Work out the finished part from the listing and answer in its coordinate system (mm). A direction names the side the tool comes from. Coordinates: 2 decimals unless noted, no trailing zeros. Order: outer loops, then holes, each group sorted by start corner. A loop starts at its lowest first (then second) coordinate and runs counter-clockwise, first axis right, second up.
1. The part is cut by section C-C, the plane x = -35.5. Give the vertices of the cut face in (y, z).
2. Determine the mould class of faces 5 (the flat face through (-2, -476.179, 214)), 6 (the flat face through (-512.899, -98, 84)), 7 (the flat face through (-12, 489, 215.9)) for opening direction Y: +Y half, -Y half, draft (parallel to the pull), parting line (faces both ways), or undercut.
3. The part is cut by section B-B, the plane z = 109. Give the vertices of the cut face in (x, y).
4. Find the intervals of material crossed by probe 1 along Y at (x, z) = (298, 173); probe 2 along Y at (x, z) = (453.5, 57); probe 3 along X at (y, z) = (373, 88.5), in increasing order.
5. Flat-ended cylindrical pins translate along their axes: pin 1 Ø5 at (x, z) = (365.5, 160) entering from +Y; pin 2 Ø3 at (x, y) = (162, 30.5) entering from -Z. Find the tip coordinate at first contact, or state that the pin passes through.
6. The part is cut by section D-D, the plane z = 12. Give the vertices of the cut face in (x, y), then the cut area to 3 significant figures.
7. The part is cut by section A-A, the plane y = 359. Give the vertices of the cut face in (x, z), then the cut area to 3 significant figures.
8. A tool of negligible diameter and unlimited length cuts with its end or side. For faces 1 (the flat face through (2, 463.621, 91)), 2 (the flat face through (-12, -399.979, 126)), 3 (the flat face through (-12, 38.171, 132)), 4 (the flat face through (-12, 25.471, 126)), from which of +Z, -Z, +X, -X, +Y, -Y can it reach the whole face along a straight path? Write none if from no direction.
```python
from build123d import *

# Parameters (mm, degrees)
SKETCH1_W            = 1016
SKETCH1_H            = 412.75
BOSS_EXTRUDE2_DEPTH  = 203.2
SKETCH3_W            = 1041.4
SKETCH3_H            = 939.8
BOSS_EXTRUDE4_DEPTH  = 25.4
SKETCH6_W            = 12.7
SKETCH6_H            = 939.8
BOSS_EXTRUDE7_DEPTH  = 50.8
SKETCH7_W            = 12.7
SKETCH7_H            = 939.8
BOSS_EXTRUDE8_DEPTH  = 50.8
BOSS_EXTRUDE9_DEPTH  = 50.8
SKETCH10_W           = 1016
SKETCH10_H           = 514.35
CUT_EXTRUDE1_DEPTH   = 50.8
SKETCH11_W           = 1016
SKETCH11_H           = 12.7
BOSS_EXTRUDE11_DEPTH = 38.1
SKETCH13_W           = 1016
SKETCH13_H           = 76.2
BOSS_EXTRUDE12_DEPTH = 12.7


with BuildPart() as part:
    # Sketch1 → Boss-Extrude2 (new body)
    with BuildSketch(Plane.XY):
        Polygon((-512.899336879, -399.978806382), (503.100663121, -399.978806382), (503.100663121, -463.478806382), (503.100663121, -476.178806382), (515.800663121, -476.178806382), (515.800663121, 463.621193618), (-525.599336879, 463.621193618), (-525.599336879, -476.178806382), (-512.899336879, -476.178806382), (-512.899336879, -463.478806382), align=None)
        with Locations((-4.899336879, 244.546193618)):
            Rectangle(SKETCH1_W, SKETCH1_H, mode=Mode.SUBTRACT)
        with Locations((-4.899336879, -180.903806382)):
            Rectangle(SKETCH1_W, SKETCH1_H, mode=Mode.SUBTRACT)
    extrude(amount=BOSS_EXTRUDE2_DEPTH)

    # Sketch3 → Boss-Extrude4 (add)
    with BuildSketch(Plane.XY.offset(203.2)):
        with Locations((-4.899336879, -6.278806382)):
            Rectangle(SKETCH3_W, SKETCH3_H)
    extrude(amount=BOSS_EXTRUDE4_DEPTH)

    # Sketch6 → Boss-Extrude7 (add)
    with BuildSketch(Plane(origin=(0, 0, 0), x_dir=(-1, 0, 0), z_dir=(0, 0, -1))):
        with Locations((-509.450663121, -6.278806382)):
            Rectangle(SKETCH6_W, SKETCH6_H)
    extrude(amount=BOSS_EXTRUDE7_DEPTH)

    # Sketch7 → Boss-Extrude8 (add)
    with BuildSketch(Plane(origin=(0, 0, 0), x_dir=(-1, 0, 0), z_dir=(0, 0, -1))):
        with Locations((519.249336879, -6.278806382)):
            Rectangle(SKETCH7_W, SKETCH7_H)
    extrude(amount=BOSS_EXTRUDE8_DEPTH)

    # Sketch8 → Boss-Extrude9 (add)
    with BuildSketch(Plane(origin=(0, 463.621193618, 0), x_dir=(1, 0, 0), z_dir=(0, 1, 0))):
        Polygon((-512.899336879, 0), (-512.899336879, -215.9), (503.100663121, -215.9), (503.100663121, 0), (503.100663121, 50.8), (515.800663121, 50.8), (515.800663121, 0), (515.800663121, -228.6), (-525.599336879, -228.6), (-525.599336879, 0), (-525.599336879, 50.8), (-512.899336879, 50.8), align=None)
    extrude(amount=BOSS_EXTRUDE9_DEPTH)

    # Sketch10 → Cut-Extrude1 (cut)
    with BuildSketch(Plane(origin=(0, 0, 0), x_dir=(-1, 0, 0), z_dir=(0, 0, -1))):
        with Locations((4.899336879, -219.003806382)):
            Rectangle(SKETCH10_W, SKETCH10_H)
    extrude(amount=-CUT_EXTRUDE1_DEPTH, mode=Mode.SUBTRACT)

    # Sketch11 → Boss-Extrude11 (add)
    with BuildSketch(Plane(origin=(0, 0, 0), x_dir=(-1, 0, 0), z_dir=(0, 0, -1))):
        with Locations((4.899336879, 457.271193618)):
            Rectangle(SKETCH11_W, SKETCH11_H)
    extrude(amount=BOSS_EXTRUDE11_DEPTH)

    # Sketch13 → Boss-Extrude12 (add)
    with BuildSketch(Plane(origin=(0, 0, 50.8), x_dir=(-1, 0, 0), z_dir=(0, 0, -1))):
        with Locations((4.899336879, 63.571193618)):
            Rectangle(SKETCH13_W, SKETCH13_H)
        with Locations((4.899336879, -361.878806382)):
            Rectangle(SKETCH13_W, SKETCH13_H)
    extrude(amount=-BOSS_EXTRUDE12_DEPTH)


solid = part.part
```
Geometry says:
1. outline: (-476.18, 203.2) - (-399.98, 203.2) - (-399.98, 50.8) - (-323.78, 50.8) - (-323.78, 63.5) - (-387.28, 63.5) - (-387.28, 203.2) - (25.47, 203.2) - (25.47, 50.8) - (101.67, 50.8) - (101.67, 63.5) - (38.17, 63.5) - (38.17, 203.2) - (450.92, 203.2) - (450.92, -38.1) - (463.62, -38.1) - (463.62, 215.9) - (514.42, 215.9) - (514.42, 228.6) - (-476.18, 228.6) - close
2. face 5: -Y half
2. face 6: undercut
2. face 7: draft
3. outline: (-525.6, -476.18) - (-512.9, -476.18) - (-512.9, -399.98) - (503.1, -399.98) - (503.1, -476.18) - (515.8, -476.18) - (515.8, 514.42) - (503.1, 514.42) - (503.1, 463.62) - (-512.9, 463.62) - (-512.9, 514.42) - (-525.6, 514.42) - close; hole (-512.9, -387.28) - (503.1, -387.28) - (503.1, 25.47) - (-512.9, 25.47) - close; hole (-512.9, 38.17) - (503.1, 38.17) - (503.1, 450.92) - (-512.9, 450.92) - close
4. probe 1: y = -399.98 to -387.28, 25.47 to 38.17, 450.92 to 463.62
4. probe 2: y = -399.98 to -323.78, 25.47 to 101.67, 450.92 to 463.62
4. probe 3: x = -525.6 to -512.9, 503.1 to 515.8
5. pin 1: stops at y = 463.62
5. pin 2: stops at z = 50.8
6. outline: (-525.6, -476.18) - (-512.9, -476.18) - (-512.9, 450.92) - (503.1, 450.92) - (503.1, -476.18) - (515.8, -476.18) - (515.8, 514.42) - (503.1, 514.42) - (503.1, 463.62) - (-512.9, 463.62) - (-512.9, 514.42) - (-525.6, 514.42) - close
6. area: 38,100 mm2
7. outline: (-525.6, -50.8) - (-512.9, -50.8) - (-512.9, 203.2) - (503.1, 203.2) - (503.1, -50.8) - (515.8, -50.8) - (515.8, 228.6) - (-525.6, 228.6) - close
7. area: 32,900 mm2
8. face 1: -Z, +Y
8. face 2: -Z, -Y
8. face 3: none
8. face 4: -Z
